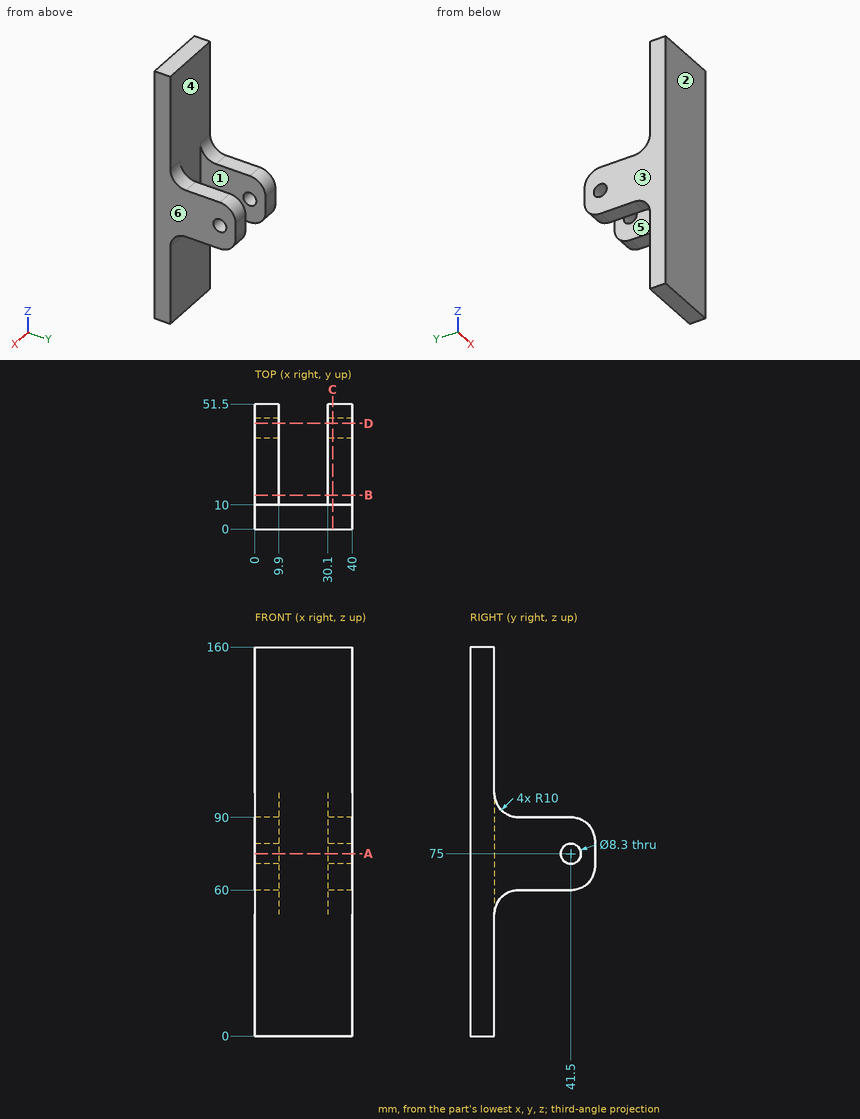
Here's the drawing with two shaded views (mm, measured from the low corner). I have some questions. A direction names the side the tool comes from. Coordinates: 2 decimals unless noted, no trailing zeros. Write each loop counter-clockwise with the first axis right and the second up, starting at its lowest first coordinate (ties: lowest second). Pieces come first, ordered by that corner, then holes. Notation, with made-up numbers: (55.5, 33) -> (76.5, 33) arc R19 cw to (76.5, 68) -> close; hole circle Ø10 at (47.5, 0.5). An arc over 180 degrees is marked (long way). Answer as CSV lines item,"result".
1) If we section it at A-A on z = 75: Please give me the cut outline in (x, y).
Check result:
outline,"(0, 0) -> (40, 0) -> (40, 37.35) -> (30.1, 37.35) -> (30.1, 10) -> (9.9, 10) -> (9.9, 37.35) -> (0, 37.35) -> close; (0, 45.65) -> (9.9, 45.65) -> (9.9, 51.5) -> (0, 51.5) -> close; (30.1, 45.65) -> (40, 45.65) -> (40, 51.5) -> (30.1, 51.5) -> close"
2) If we section it at C-C on x = 32: Please give me the cut outline in (y, z), then the cut area to 3 significant figures.
Check result:
outline,"(0, 0) -> (10, 0) -> (10, 50) arc R10 cw to (20, 60) -> (41.5, 60) arc R10 ccw to (51.5, 70) -> (51.5, 80) arc R10 ccw to (41.5, 90) -> (20, 90) arc R10 cw to (10, 100) -> (10, 160) -> (0, 160) -> close; hole circle Ø8.3 at (41.5, 75)"
area,"2,790 mm²"
3) If we mould it in two halves opening along X, with no side actions, what happens to the marked faces 1, 2 and 3? For each: +X half, -X half, draft (parallel to the pull), parting line (faces both ways), or undercut.
Check result:
face 1,"undercut"
face 2,"draft"
face 3,"-X half"
4) If I drill on line 1 (Z direction, x = 35, y = 41); line 2 (X direction, y = 11, z = 88); line 3 (Y direction, x = 7.75, z = 75), over which ranges is the centre line in solid material (lowest first)? Write a range as from..to.
Check result:
line 1,"60..70.88, 79.12..90"
line 2,"0..9.9, 30.1..40"
line 3,"0..37.35, 45.65..51.5"
5) On a 3-axis mill with a long thin cutter (end or side, diameter ignored), from which of +Z, -Z, +X, -X, +Y, -Y can I reach the whole of each face in a straight line? I mean the marked faces 4, 5 and 6. Say none if no direction works.
Check result:
face 4,"+Y"
face 5,"+Z, -Z, +Y"
face 6,"+Z, -Z, +X, +Y, -Y"
6) If we section it at B-B on y = 14: Please give me the cut outline in (x, z), then the cut area to 3 significant figures.
Check result:
outline,"(0, 58) -> (9.9, 58) -> (9.9, 92) -> (0, 92) -> close; (30.1, 58) -> (40, 58) -> (40, 92) -> (30.1, 92) -> close"
area,"673 mm²"
7) If we section it at D-D on y = 43.5: Please give me the cut outline in (x, z), then the cut area to 3 significant figures.
Check result:
outline,"(0, 60.2) -> (9.9, 60.2) -> (9.9, 71.36) -> (0, 71.36) -> close; (0, 78.64) -> (9.9, 78.64) -> (9.9, 89.8) -> (0, 89.8) -> close; (30.1, 60.2) -> (40, 60.2) -> (40, 71.36) -> (30.1, 71.36) -> close; (30.1, 78.64) -> (40, 78.64) -> (40, 89.8) -> (30.1, 89.8) -> close"
area,"442 mm²"
8) Will these pins go through, and if not, where does the flat tip stop? P1, Ø4, axis at x = 29.5, y = 33.5, coming from the -Z side; P2, Ø8, axis at x = 33, y = 26, coming from the +Z side; P3, Ø1, axis at x = 15.5, z = 98, coming from the +Y side; P4, Ø4, axis at x = 31.5, z = 44, coming from the -Y side.
Check result:
P1,"z = 60"
P2,"z = 90"
P3,"y = 10"
P4,"y = 0"
